Verification items for the finished model (mm, model axes). A direction names the side the tool comes from. Give positions to 0.01 mm unless a question says otherwise; leave off trailing zeros. Loops run counter-clockwise (first coordinate to the right, second up) from the corner with the lowest first, then second, coordinate; pieces in that order, holes last. Notation, with made-up numbers: (-26, 56) - (22, 56) arc R26 cw to (22, 74) - close; hole circle Ø7 at (64, 89). An arc over 180 degrees is marked (long way). One line per question, with ' | ' between items. Start each with the question number.
1. Depth check by flat-ended pin: pin 1 Ø10 at (x, y) = (80.5, 3.5) entering from -Z; pin 2 Ø1 at (x, y) = (41, 10.5) entering from +Z; pin 3 Ø12 at (x, z) = (35, 9) entering from -Y. Enter the tip coordinate at first touch or a pass-through.
2. Section check B-B, the plane z = 0. Enter the section's corners in (x, y).
3. Tool access check on faces 1 (the face through (50.314, 12.932, -5.362)), 2 (the face through (12.77, -1.15, 16.37)), 3 (the face through (12.77, -16.37, -1.15)). Record the directions out of +Z, -Z, +X, -X, +Y, -Y that give a thin tool (end or side, any length) a straight path to the whole face; none if there is none.
4. Section check C-C, the plane x = 10. Enter the section's corners in (y, z), then the cut area to 3 significant figures.
5. Thickness scan on line 1 along Z through (x, y) = (79, 0); line 2 along X through (y, z) = (0, 16.1). Record the ranges inside material, lowest first. Write a range as from..to.
6. Section check D-D, the plane x = 47. Enter the section's corners in (y, z), then the cut area to 3 significant figures.
7. Section check A-A, the plane y = 0. Enter the section's corners in (x, z).
8. Mould release check, pull along Y, two halves, no side actions. Record for faces 4 (the face through (100, -9, -11)), 5 (the face through (1.875, 13.473, 4.243)), 6 (the face through (49.3, 8.767, -16.856)): +Y half, -Y half, draft (parallel to the pull), parting line (faces both ways), or undercut.
from build123d import *

# Parameters (mm, degrees)
F0_R     = 19
F0_R_2   = 14
F1_DEPTH = 100
F2_SIZE2 = 2
F2_SIZE  = 2
F5_R     = 3
F6_DEPTH = 5.3262057688
F7_R     = 3
F8_DEPTH = 5.3262057688


with BuildPart() as f1:
    # F0 (on Right) → F1 (new body)
    with BuildSketch(Plane.YZ):
        Circle(F0_R)
        Circle(F0_R_2, mode=Mode.SUBTRACT)
    extrude(amount=F1_DEPTH)

    # F2
    f2_edges = [f1.edges().sort_by_distance(p)[0] for p in [
        (0, -14, 0),
    ]]
    chamfer(f2_edges, length=F2_SIZE, length2=F2_SIZE2)

    # F5 (on offset) → F6 (cut, through all)
    with BuildSketch(Plane.XY.offset(19)):
        with Locations((10, 0)):
            Circle(F5_R)
    extrude(amount=-F6_DEPTH, mode=Mode.SUBTRACT)

    # F7 (on offset) → F8 (cut, through all)
    with BuildSketch(Plane.XZ.offset(19)):
        with Locations((10, 0)):
            Circle(F7_R)
    extrude(amount=-F8_DEPTH, mode=Mode.SUBTRACT)


solid = f1.part
Results list:
1) pin 1: z = -19 | pin 2: z = 16.16 | pin 3: y = -18.76
2) outline: (0, -19) - (7, -19) - (7, -14) - (2, -14) - (0, -16) - close; (0, 16) - (2, 14) - (100, 14) - (100, 19) - (0, 19) - close; (13, -19) - (100, -19) - (100, -14) - (13, -14) - close
3) face 1: +X, -X | face 2: +Z | face 3: -Y
4) outline: (-18.76, -3) arc R19 ccw (long way) to (3, 18.76) - (3, 13.67) arc R14 cw (long way) to (-13.67, -3) - close; (-18.76, 3) - (-13.67, 3) arc R14 cw to (-3, 13.67) - (-3, 18.76) arc R19 ccw to start | area: 458 mm²
5) line 1: -19..-14, 14..19 | line 2: 0..7, 13..100
6) outline: circle Ø38 at (0, 0); hole circle Ø28 at (0, 0) | area: 518 mm²
7) outline: (0, -19) - (100, -19) - (100, -14) - (2, -14) - (0, -16) - close; (0, 16) - (2, 14) - (7, 14) - (7, 19) - (0, 19) - close; (13, 14) - (100, 14) - (100, 19) - (13, 19) - close
8) face 4: draft | face 5: undercut | face 6: parting line
